```python
from build123d import *

# Parameters (mm, degrees)
THREAD1_PITCH = 2


with BuildPart() as part:
    # Sketch1 → Revolve1 (revolve)
    with BuildSketch(Plane(origin=(0, 0, 0), x_dir=(0, 0, -1), z_dir=(1, 0, 0))):
        Polygon((-7.5, 2.5), (-7.5, -4), (-10, -4), (-10, 4), (-7.5, 4), (-7.5, 9), (-5.75, 9), (-5.75, 2.5), align=None)
    revolve(axis=Axis((0, 15.090909091, 0), (0, -1, 0)))

    # Thread1: the profile of Thread Profile1 profile screwed along a right-hand helix of 5 turns, 10 arcs to a turn; built about Z, then put on its axis
    thread1_z = Axis((0, 0, 0), (0, 0, 1))
    thread1_corners = [(7.4997, 0, -0.000173205), (8.58253175, 0, 0.624999997), (8.58253175, 0, 0.874999997), (7.4997, 0, 1.5001732)]
    with BuildLine(mode=Mode.PRIVATE) as thread1_profile:
        Line(thread1_corners[0], thread1_corners[1])
        Line(thread1_corners[1], thread1_corners[2])
        Line(thread1_corners[2], thread1_corners[3])
        Line(thread1_corners[3], thread1_corners[0])
    thread1_cap = Face(thread1_profile.wire())
    thread1_turn_angles = [0, 18, 36, 54, 72, 90, 108, 126, 144, 162, 180, 198, 216, 234, 252, 270, 288, 306, 324, 342, 360]
    thread1_turn_weights = [1, 0.9510565162951535, 1, 0.9510565162951535, 1, 0.9510565162951535, 1, 0.9510565162951535, 1, 0.9510565162951535, 1, 0.9510565162951535, 1, 0.9510565162951535, 1, 0.9510565162951535, 1, 0.9510565162951535, 1, 0.9510565162951535, 1]
    thread1_turn_rails = [Edge.make_bspline([Vector(p[0], p[1], 0).rotate(thread1_z, thread1_turn_angles[k]) / thread1_turn_weights[k] + Vector(0, 0, p[2] + THREAD1_PITCH * thread1_turn_angles[k] / 360) for k in range(21)], [0, 0, 0, 1, 1, 2, 2, 3, 3, 4, 4, 5, 5, 6, 6, 7, 7, 8, 8, 9, 9, 10, 10, 10], 2, thread1_turn_weights) for p in thread1_corners]
    thread1_turn_sides = [Face.make_surface_from_curves(thread1_turn_rails[p[0]], thread1_turn_rails[p[1]]) for p in [(0, 1), (1, 2), (2, 3), (3, 0)]]
    thread1 = Plane(origin=(0, -9, 0), x_dir=(1, 0, 0), z_dir=(0, 1, 0)) * Solid(Shell([*[p.moved(Location((0, 0, THREAD1_PITCH * i))) for i in range(5) for p in thread1_turn_sides], thread1_cap, thread1_cap.rotate(thread1_z, 1800).moved(Location((0, 0, THREAD1_PITCH * 1800 / 360)))]))
    add(thread1, mode=Mode.SUBTRACT)


solid = part.part
```
Verification items for the finished model (mm, model axes). Round coordinates to 2 decimals unless told otherwise and drop trailing zeros. Write each loop counter-clockwise with the first axis right and the second up, starting at its lowest first coordinate (ties: lowest second). Pieces come first, ordered by that corner, then holes.
1. Gauge pin test, flat ends, axial feed: P1, Ø1.5, axis at y = 7.5, z = -2, coming from the +X side; P2, Ø0.9, axis at x = 8.5, y = 1.5, coming from the +Z side; P3, Ø3, axis at x = -6, y = 1.5, coming from the -Z side. Record the tip position at first contact, or that the pin passes through.
2. Draft check along Y on faces 1 (the flat face through (-7, 4, 4)), 2 (the cylindrical face through (-0.33, 6.535, -7.493)), 3 (the flat face through (6, 2.5, 2)), 4 (the flat face through (8, 2, 0)). Enter one of: +Y half, -Y half, draft (parallel to the pull), parting line (faces both ways), or undercut.
3. Scan lines: L1, parallel to X at y = 4.25, z = 0; L2, parallel to Y at x = -7, z = 4; L3, parallel to Z at x = 0, y = 1.4. Record each from-to range of solid material in increasing order.
4. Section check A-A on y = 4.5. Enter the section's corners in (x, z).
Answer:
1. P1: stops at x = 7.4
1. P2: stops at z = 5.93
1. P3: stops at z = -8.93
2. face 1: +Y half
2. face 2: draft
2. face 3: -Y half
2. face 4: undercut
3. L1: x = -7.5 to -5.75, 5.75 to 7.5
3. L2: y = -4 to -3.51, -2.66 to -1.51, -0.66 to 0.49, 1.34 to 4
3. L3: z = -10 to -7.5, 8.54 to 10
4. outline: circle Ø15 at (0, 0); hole circle Ø11.5 at (0, 0)
